Source: CAD feature listing. Evaluate the final solid. Frame: model axes, mm. A direction names the side the tool comes from. Give positions to 0.01 mm unless a question says otherwise; leave off trailing zeros. Write each loop counter-clockwise with the first axis right and the second up, starting at its lowest first coordinate (ties: lowest second). Pieces come first, ordered by that corner, then holes. Notation, with made-up numbers: M 82,-4 L 86,-4 A33 ccw 86,32 Z; hole C 75.5,88.25 d5. An arc over 180 degrees is marked long. Return JSON: item names as keys, results as strings.
```python
from build123d import *

# Parameters (mm, degrees)
SKETCH_1_W      = 20
SKETCH_1_H      = 20
SKETCH_1_R      = 1.5
EXTRUDE_1_DEPTH = 2
SKETCH_2_R      = 7
SKETCH_2_R_2    = 5
EXTRUDE_2_DEPTH = 3


with BuildPart() as part:
    # 草图1 → 凸台-拉伸1 (new body)
    with BuildSketch(Plane.XY):
        Rectangle(SKETCH_1_W, SKETCH_1_H)
        with Locations((-7, 7)):
            Circle(SKETCH_1_R, mode=Mode.SUBTRACT)
        with Locations((7, 7)):
            Circle(SKETCH_1_R, mode=Mode.SUBTRACT)
        with Locations((7, -7)):
            Circle(SKETCH_1_R, mode=Mode.SUBTRACT)
        with Locations((-7, -7)):
            Circle(SKETCH_1_R, mode=Mode.SUBTRACT)
    extrude(amount=EXTRUDE_1_DEPTH)

    # 草图2 → 凸台-拉伸2 (add)
    with BuildSketch(Plane.XY.offset(2)):
        Circle(SKETCH_2_R)
        Circle(SKETCH_2_R_2, mode=Mode.SUBTRACT)
    extrude(amount=EXTRUDE_2_DEPTH)


solid = part.part
```
1) Draft query along X for faces 3 (the face through (6.466, -2.681, 3.479)), 4 (the face through (-8.2, -7.9, 1)), 5 (the face through (0, 10, 1)). Return one class per face: released by +X, released by -X, zero draft, split by the parting line, or undercut.
Numbers:
{"face 3": "split by the parting line", "face 4": "undercut", "face 5": "zero draft"}
2) Cut plane A-A, the plane z = 0.7. Return the cut outline in (x, y), then the cut area to 3 significant figures.
Numbers:
{"outline": "M -10,-10 L 10,-10 L 10,10 L -10,10 Z; hole C -7,-7 d3; hole C -7,7 d3; hole C 7,-7 d3; hole C 7,7 d3", "area": "372 mm²"}
3) Line query: line 1 (Y direction, x = 7, z = 1.1); line 2 (Y direction, x = 0, z = 4.05); line 3 (Y direction, x = -8, z = 1.65). Output: solid intervals per line, ascending. Write a range as [from, to].
Numbers:
{"line 1": "y = [-10, -8.5], [-5.5, 5.5], [8.5, 10]", "line 2": "y = [-7, -5], [5, 7]", "line 3": "y = [-10, -8.12], [-5.88, 5.88], [8.12, 10]"}
4) Contact query for flat-ended pins moving along their axis: pin 1 Ø3.5 at (x, y) = (7, -7) entering from +Z; pin 2 Ø2.5 at (x, y) = (7, 7) entering from +Z. Output: stop coordinate, or through.
Numbers:
{"pin 1": "stops at z = 2", "pin 2": "passes through"}
5) Cut plane D-D, the plane x = -4.75. Return the cut outline in (y, z).
Numbers:
{"outline": "M -10,0 L 10,0 L 10,2 L 5.14,2 L 5.14,5 L 1.56,5 L 1.56,2 L -1.56,2 L -1.56,5 L -5.14,5 L -5.14,2 L -10,2 Z"}
6) Cut plane C-C, the plane x = 6.75. Return the cut outline in (y, z).
Numbers:
{"outline": "M -10,0 L -8.48,0 L -8.48,2 L -10,2 Z; M -5.52,0 L 5.52,0 L 5.52,2 L 1.85,2 L 1.85,5 L -1.85,5 L -1.85,2 L -5.52,2 Z; M 8.48,0 L 10,0 L 10,2 L 8.48,2 Z"}
7) Cut plane B-B, the plane y = -6.5. Return the cut outline in (x, z), then the cut area to 3 significant figures.
Numbers:
{"outline": "M -10,0 L -8.41,0 L -8.41,2 L -10,2 Z; M -5.59,0 L 5.59,0 L 5.59,2 L 2.6,2 L 2.6,5 L -2.6,5 L -2.6,2 L -5.59,2 Z; M 8.41,0 L 10,0 L 10,2 L 8.41,2 Z", "area": "44.3 mm²"}
8) Set-up query: faces 1 (the face through (-8.2, 6.1, 1)), 2 (the face through (0, 0, 2)). Return all of +Z, -Z, +X, -X, +Y, -Y with unobstructed straight access to the full face (end or side cutting, diameter ignored); none if empty.
Numbers:
{"face 1": "+Z, -Z", "face 2": "+Z"}
